Verification items for this drawing (mm, ordinates from the low corner). A direction names the side the tool comes from. Round coordinates to 2 decimals unless told otherwise and drop trailing zeros. Order: outer loops, then holes, each group sorted by start corner. A loop starts at its lowest first (then second) coordinate and runs counter-clockwise, first axis right, second up. Notation, with made-up numbers: M -36,2.5 L -28,2.5 A19 ccw -28,7.5 Z; hole C 57,9.25 d10. An arc over 180 degrees is marked long. Use CSV: the item, a comma, the result in double quotes. Start each with the question number.
Q1. Sectioned sample at C-C (x = 7.5). Enter the section's corners in (y, z), and give its area (3 significant figures).
Q2. Set-up check for the marked faces 1 and 2: record each of +Z, -Z, +X, -X, +Y, -Y from which the full face is reachable in a straight line by a thin tool's end or side.
Q3. Mould release check, pull along X, two halves, no side actions. Record for the marked faces 3, 4, 5 and 6: +X half, -X half, draft (parallel to the pull), parting line (faces both ways), or undercut.
Q4. Sectioned sample at B-B (y = 20). Enter the section's corners in (x, z), and give its area (3 significant figures).
Q5. Sectioned sample at D-D (z = 7.5). Enter the section's corners in (x, y), and give its area (3 significant figures).
Q6. Sectioned sample at A-A (z = 23). Enter the section's corners in (x, y).
Q7. Gauge pin test, flat ends, axial feed: pin 1 Ø3 at (x, z) = (38.5, 38.5) entering from +Y; pin 2 Ø5 at (x, y) = (6.5, 11.5) entering from +Z; pin 3 Ø6 at (x, z) = (24.5, 39) entering from +Y. Record the tip position at first contact, or that the pin passes through.
Q8. Scan lines: line 1 (Z direction, x = 38.5, y = 1.55); line 2 (X direction, y = 12, z = 9.5); line 3 (Z direction, x = 23, y = 0.6). Record each from-to range of solid material in increasing order.
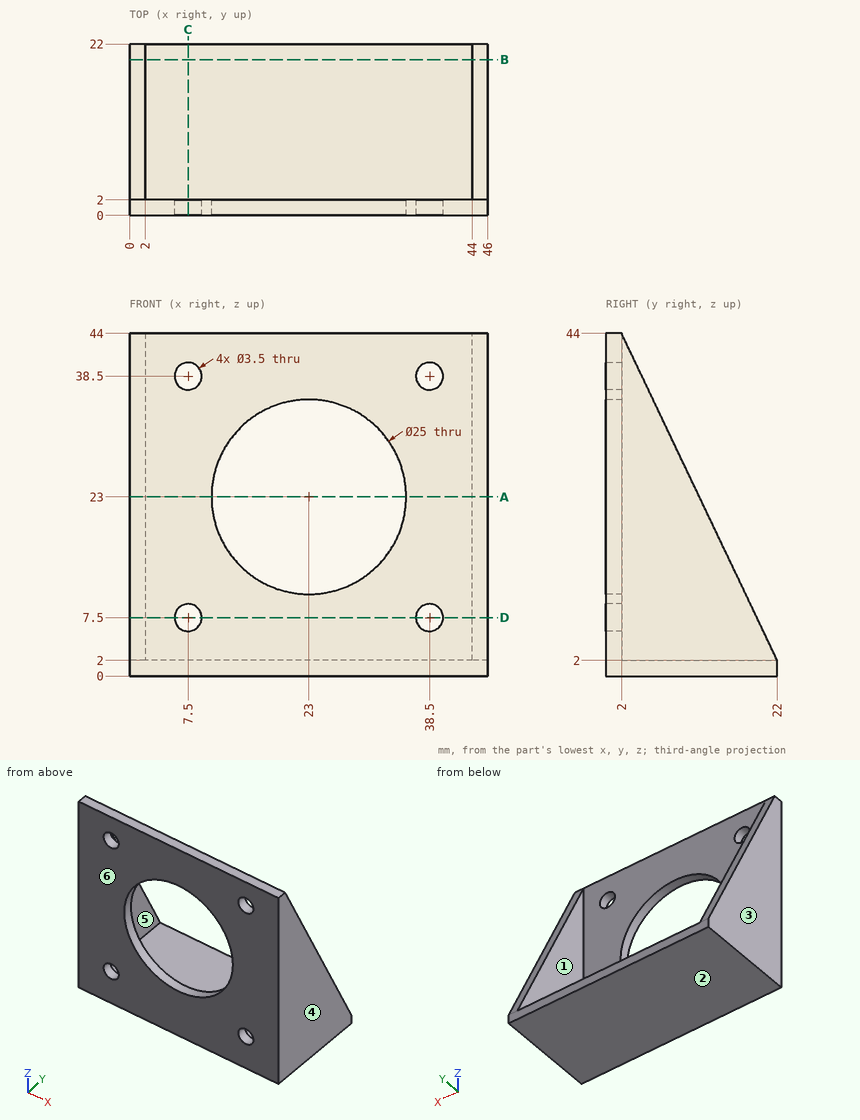
Verdict:
1,outline,"M 0,0 L 22,0 L 22,2 L 2,2 L 2,5.75 L 0,5.75 Z; M 0,9.25 L 2,9.25 L 2,36.75 L 0,36.75 Z; M 0,40.25 L 2,40.25 L 2,44 L 0,44 Z"
1,area,"114 mm²"
2,face 1,"+Z, +Y"
2,face 2,"-Z, +X, -X, +Y, -Y"
3,face 3,"-X half"
3,face 4,"+X half"
3,face 5,"undercut"
3,face 6,"draft"
4,outline,"M 0,0 L 46,0 L 46,6.2 L 44,6.2 L 44,2 L 2,2 L 2,6.2 L 0,6.2 Z"
4,area,"109 mm²"
5,outline,"M 0,0 L 5.75,0 L 5.75,2 L 2,2 L 2,19.38 L 0,19.38 Z; M 9.25,0 L 36.75,0 L 36.75,2 L 9.25,2 Z; M 40.25,0 L 46,0 L 46,19.38 L 44,19.38 L 44,2 L 40.25,2 Z"
5,area,"148 mm²"
6,outline,"M 0,0 L 10.5,0 L 10.5,2 L 2,2 L 2,12 L 0,12 Z; M 35.5,0 L 46,0 L 46,12 L 44,12 L 44,2 L 35.5,2 Z"
7,pin 1,"passes through"
7,pin 2,"stops at z = 2"
7,pin 3,"stops at y = 2"
8,line 1,"z = 0 to 5.75, 9.25 to 36.75, 40.25 to 44"
8,line 2,"x = 0 to 2, 44 to 46"
8,line 3,"z = 0 to 10.5, 35.5 to 44"
